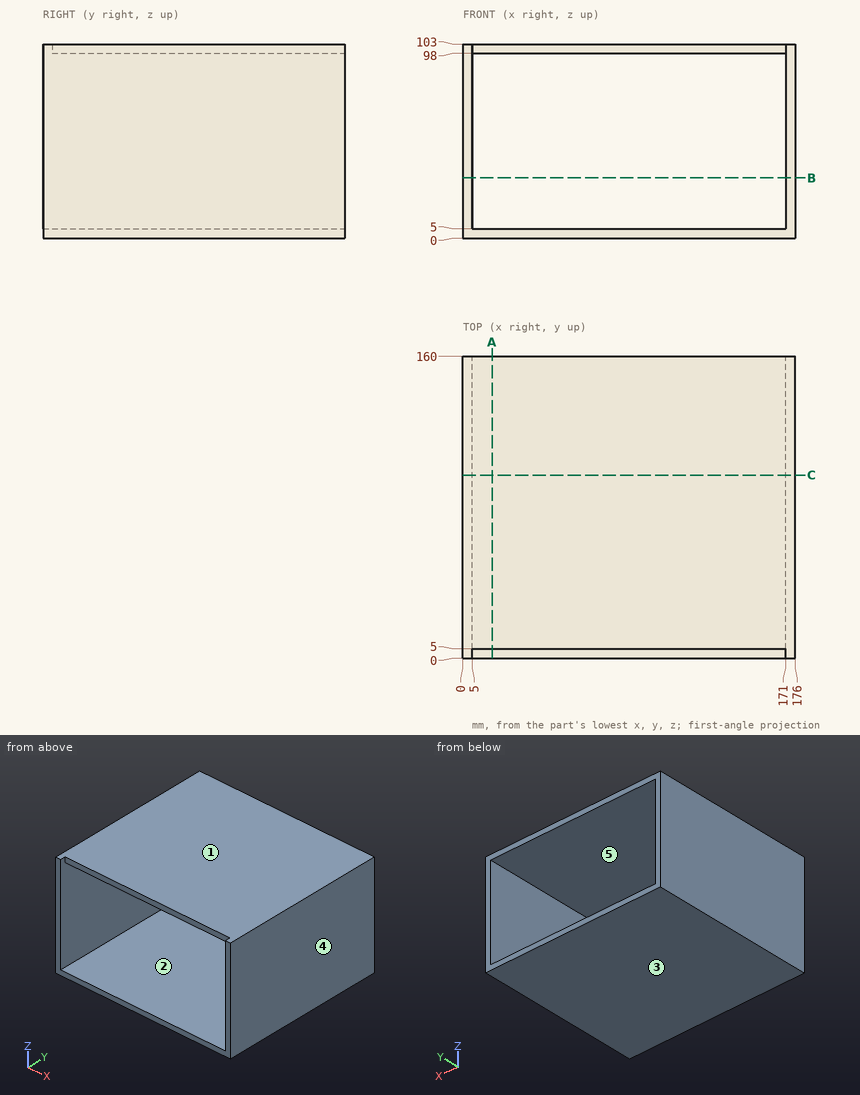
Can you work these out from the drawing? Everything is in mm from the part's minimum corner. A direction names the side the tool comes from. Coordinates: 2 decimals unless noted, no trailing zeros. Loops run counter-clockwise (first coordinate to the right, second up) from the corner with the lowest first, then second, coordinate; pieces in that order, holes last. Notation, with made-up numbers: M 70,-9 L 120,-9 A28 cw 120,30 Z; hole C 88.25,8 d6. An arc over 180 degrees is marked long. Put each result on its own line as item: value. Start each with the question number.
(1) Suppose I cut it at C-C on y = 97. Please give me the cut outline in (x, z), then the cut area to 3 significant figures.
(2) I need wall thicknesses on line 1 (X direction, y = 112, z = 88); line 2 (Z direction, x = 65, y = 16.5); line 3 (Y direction, x = 117, z = 98.5). Which ranges of each line are inside material? Lowest first, please. Write a range as from..to.
(3) Will these pins go through, and if not, where does the flat tip stop? P1, Ø1.5, axis at x = 111, z = 99.5, coming from the -Y side; P2, Ø6, axis at y = 51.5, z = 18, coming from the -X side.
(4) Thinking about a two-plate mould opening in Z: for the marked faces 3, 4 and 5, which applies, pulls with the +Z half, pulls with the -Z half, needs draft (parallel to the pull), parting line crosses it, or undercut?
(5) Suppose I cut it at A-A on x = 15.5. Please give me the cut outline in (y, z).
(6) For the marked faces 1 and 2, which set-ups out of +Z, -Z, +X, -X, +Y, -Y let a thin tool reach every point of the face, with its end or its side?
(7) Suppose I cut it at B-B on z = 32. Please give me the cut outline in (x, y).
Solutions:
1. outline: M 0,0 L 176,0 L 176,103 L 0,103 Z; hole M 5,5 L 171,5 L 171,98 L 5,98 Z
1. area: 2,690 mm2
2. line 1: x = 0..5, 171..176
2. line 2: z = 0..5, 98..103
2. line 3: y = 5..160
3. P1: stops at y = 5
3. P2: stops at x = 0
4. face 3: pulls with the -Z half
4. face 4: needs draft
4. face 5: undercut
5. outline: M 0,0 L 160,0 L 160,5 L 0,5 Z; M 5,98 L 160,98 L 160,103 L 5,103 Z
6. face 1: +Z, +X, -X, +Y, -Y
6. face 2: +Y, -Y
7. outline: M 0,0 L 5,0 L 5,160 L 0,160 Z; M 171,0 L 176,0 L 176,160 L 171,160 Z
